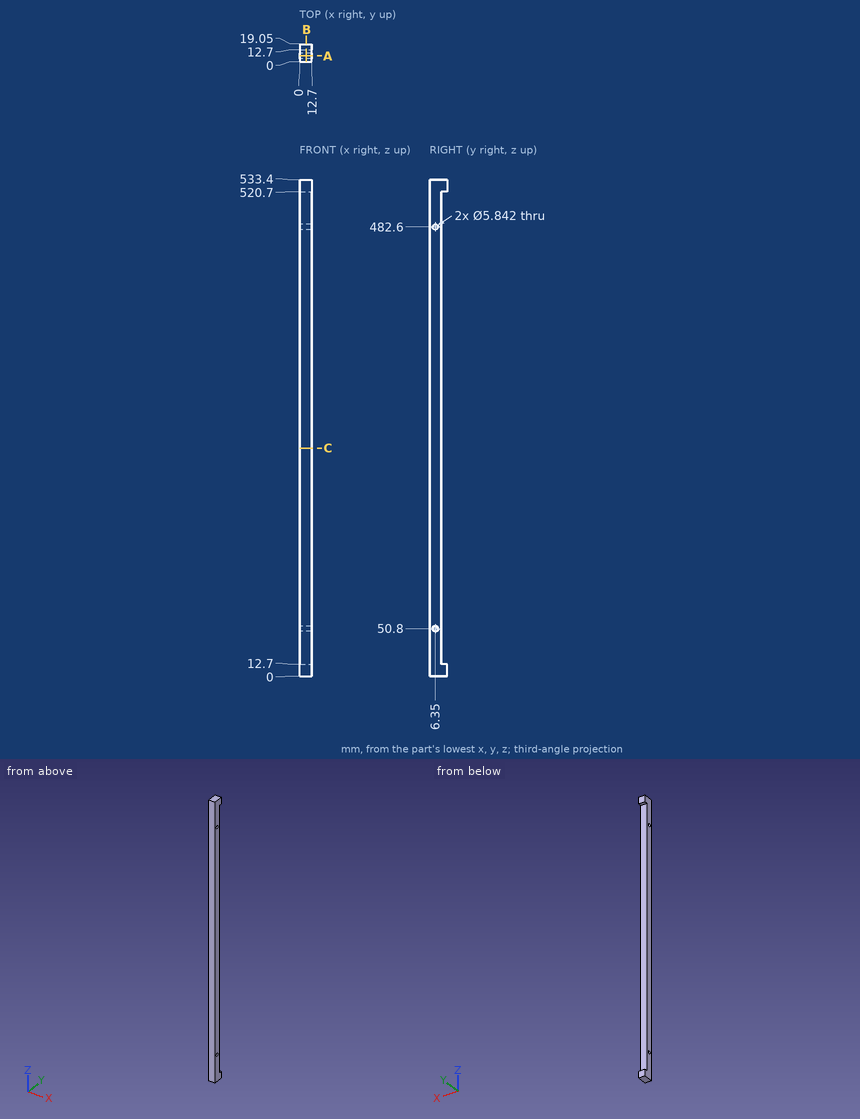
Verification items for this drawing (mm, ordinates from the low corner). Coordinates: 2 decimals unless noted, no trailing zeros. Order: outer loops, then holes, each group sorted by start corner. A loop starts at its lowest first (then second) coordinate and runs counter-clockwise, first axis right, second up. Notation, with made-up numbers: M -18.75,-31.5 L 5.25,-31.5 A24 cw 5.25,5.5 Z; hole C -21,-7.75 d10. An arc over 180 degrees is marked long. Answer as a JSON object with one key per item and string values.
Q1. Depth check by flat-ended pin: pin 1 Ø1 at (x, z) = (9.5, 226.5) entering from +Y. Enter the tip coordinate at first touch or a pass-through.
Results are:
{"pin 1": "stops at y = 12.7"}
Q2. Scan lines: line 1 (Z direction, x = 8, y = 6.35); line 2 (Z direction, x = 6.75, y = 8); line 3 (Y direction, x = 6.25, z = 50.8). Record each from-to range of solid material in increasing order.
Results are:
{"line 1": "z = 0 to 47.88, 53.72 to 479.68, 485.52 to 533.4", "line 2": "z = 0 to 48.39, 53.21 to 480.19, 485.01 to 533.4", "line 3": "y = 0 to 3.43, 9.27 to 12.7"}
Q3. Cross-section at A-A on y = 6.35. Record the cut outline in (x, z).
Results are:
{"outline": "M 0,0 L 12.7,0 L 12.7,47.88 L 0,47.88 Z; M 0,53.72 L 12.7,53.72 L 12.7,479.68 L 0,479.68 Z; M 0,485.52 L 12.7,485.52 L 12.7,533.4 L 0,533.4 Z"}
Q4. Cross-section at C-C on z = 245. Record the cut outline in (x, y), and give its area (3 significant figures).
Results are:
{"outline": "M 0,0 L 12.7,0 L 12.7,12.7 L 0,12.7 Z", "area": "161 mm²"}
Q5. Cross-section at B-B on x = 7.25. Record the cut outline in (y, z), and give its area (3 significant figures).
Results are:
{"outline": "M 0,0 L 19.05,0 L 19.05,12.7 L 12.7,12.7 L 12.7,520.7 L 19.05,520.7 L 19.05,533.4 L 0,533.4 Z; hole C 6.35,50.8 d5.84; hole C 6.35,482.6 d5.84", "area": "6,880 mm²"}
